CAD build for the part. Positions are in the model's coordinates, mm. Coordinates: 2 decimals unless noted, no trailing zeros. Loops run counter-clockwise (first coordinate to the right, second up) from the corner with the lowest first, then second, coordinate; pieces in that order, holes last. Notation, with made-up numbers: (-38, 5.5) -> (-34, 5.5) arc R29 cw to (-34, 31.5) -> close; hole circle Ø9 at (15.5, -5). An arc over 180 degrees is marked (long way). Write item = value, one per line. Start each with the question number.
(1) Band-saw the part on A-A (z = 0.8). Count the separate pieces of the cut face and the enclosed holes in it, and give its area (3 significant figures).
(2) Band-saw the part on C-C (x = 29). Write the cut outline in (y, z).
(3) Flat gauge pin, fed straight in: P1, Ø3, axis at x = -62, y = 55.5, coming from the +Z side. Where does the tip first touch, or does it go through?
(4) Drill centre lines: line 1 (X direction, y = 93.5, z = 0.4); line 2 (X direction, y = 171, z = 0.9). Where is each one in solid material? Low to high. Write a range as from..to.
(5) Band-saw the part on B-B (y = 91). Write the cut outline in (x, z), and give its area (3 significant figures).
(6) Pull direction X, two halves, no side cores. Call faces 1 (the face through (-1, 71, 0)), 2 (the face through (-43.692, 120.593, 1.479)), 3 (the face through (-63.7, 55.57, 1.48)): +X half, -X half, draft (parallel to the pull), parting line (faces both ways), or undercut.
```python
from build123d import *

# Parameters (mm, degrees)
BOSS_EXTRUDE1_DEPTH  = 3
M3_CLEARANCE_HOLE1_D = 3.4


with BuildPart() as part:
    # Sketch1 → Boss-Extrude1 (new body)
    with BuildSketch(Plane.XY):
        Polygon((0, 180), (22, 180), (66, 59.5), (66, 0), (0, 0), align=None)
    boss_extrude1 = extrude(amount=BOSS_EXTRUDE1_DEPTH)

    # M3 Clearance Hole1 (through all)
    with Locations(Plane.XY.offset(3)):
        with Locations((48, 55.5), (62, 55.5), (48, 4), (62, 4)):
            m3_clearance_hole1 = Hole(M3_CLEARANCE_HOLE1_D / 2)

    # Mirror1: Boss-Extrude1, M3 Clearance Hole1 across plane
    add(boss_extrude1.mirror(Plane(origin=(0, 180, 3), x_dir=(0, 0, 1), z_dir=(1, 0, 0))))
    add(m3_clearance_hole1.mirror(Plane(origin=(0, 180, 3), x_dir=(0, 0, 1), z_dir=(1, 0, 0))), mode=Mode.SUBTRACT)


solid = part.part
```
Findings below:
q1.separate_pieces = 1
q1.enclosed_holes = 8
q1.area = 18,400 mm²
q2.outline = (0, 0) -> (160.83, 0) -> (160.83, 3) -> (0, 3) -> close
q3.P1 = through
q4.line_1 = -53.59..53.59
q4.line_2 = -25.29..25.29
q5.outline = (-54.5, 0) -> (54.5, 0) -> (54.5, 3) -> (-54.5, 3) -> close
q5.area = 327 mm²
q6.face_1 = draft
q6.face_2 = -X half
q6.face_3 = undercut
